from build123d import *

# Parameters (mm, degrees)
SKETCH_1_W           = 30
SKETCH_1_H           = 25
SKETCH_1_W_2         = 26
SKETCH_1_H_2         = 21
EXTRUDE_1_DEPTH      = 510
CUT_EXTRUDE_4_REACH  = 512.833
SKETCH_7_R           = 2.05
CUT_EXTRUDE_7_DEPTH  = 512.03449003
SKETCH_9_R           = 2.05
CUT_EXTRUDE_9_DEPTH  = 10
SKETCH_10_R          = 4
CUT_EXTRUDE_10_DEPTH = 10
SKETCH_11_R          = 2.05
CUT_EXTRUDE_11_DEPTH = 52
SKETCH_12_W          = 15
SKETCH_12_H          = 25
CUT_EXTRUDE_12_DEPTH = 512.03449003
CUT_EXTRUDE_13_REACH = 512.833
SKETCH_5_R           = 1.55


with BuildPart() as part:
    # 草图1 → 凸台-拉伸1 (new body)
    with BuildSketch(Plane.XY):
        Rectangle(SKETCH_1_W, SKETCH_1_H)
        Rectangle(SKETCH_1_W_2, SKETCH_1_H_2, mode=Mode.SUBTRACT)
    extrude(amount=EXTRUDE_1_DEPTH)

    # 草图4 → 切除-拉伸4 (cut, up to next)
    with BuildSketch(Plane.XZ.offset(12.5), mode=Mode.PRIVATE) as cut_extrude_4_sk1:
        with BuildLine():
            Line((-7.5, 40), (-7.5, 60))
            ThreePointArc((-7.5, 60), (0, 67.5), (7.5, 60))
            Line((7.5, 60), (7.5, 40))
            ThreePointArc((7.5, 40), (0, 32.5), (-7.5, 40))
        make_face()
    cut_extrude_4_tool1 = extrude(cut_extrude_4_sk1.sketch, amount=-CUT_EXTRUDE_4_REACH, mode=Mode.PRIVATE) & part.part
    # 草图4 → 切除-拉伸4 (cut, up to next)
    with BuildSketch(Plane.XZ.offset(12.5), mode=Mode.PRIVATE) as cut_extrude_4_sk2:
        with BuildLine():
            Line((-7.5, 190), (-7.5, 210))
            ThreePointArc((-7.5, 210), (0, 217.5), (7.5, 210))
            Line((7.5, 210), (7.5, 190))
            ThreePointArc((7.5, 190), (0, 182.5), (-7.5, 190))
        make_face()
    cut_extrude_4_tool2 = extrude(cut_extrude_4_sk2.sketch, amount=-CUT_EXTRUDE_4_REACH, mode=Mode.PRIVATE) & part.part
    # 草图4 → 切除-拉伸4 (cut, up to next)
    with BuildSketch(Plane.XZ.offset(12.5), mode=Mode.PRIVATE) as cut_extrude_4_sk3:
        with BuildLine():
            Line((-7.5, 340), (-7.5, 360))
            ThreePointArc((-7.5, 360), (0, 367.5), (7.5, 360))
            Line((7.5, 360), (7.5, 340))
            ThreePointArc((7.5, 340), (0, 332.5), (-7.5, 340))
        make_face()
    cut_extrude_4_tool3 = extrude(cut_extrude_4_sk3.sketch, amount=-CUT_EXTRUDE_4_REACH, mode=Mode.PRIVATE) & part.part
    add(cut_extrude_4_tool1.solids().sort_by_distance((0, -12.5, 50))[0], mode=Mode.SUBTRACT)
    add(cut_extrude_4_tool2.solids().sort_by_distance((0, -12.5, 200))[0], mode=Mode.SUBTRACT)
    add(cut_extrude_4_tool3.solids().sort_by_distance((0, -12.5, 350))[0], mode=Mode.SUBTRACT)

    # 草图7 → 切除-拉伸7 (cut, through all)
    with BuildSketch(Plane(origin=(15, 0, 0), x_dir=(0, 0, -1), z_dir=(1, 0, 0))):
        with Locations((-30, -5.5)):
            Circle(SKETCH_7_R)
        with Locations((-50, 4.5)):
            Circle(SKETCH_7_R)
        with Locations((-70, -5.5)):
            Circle(SKETCH_7_R)
    extrude(amount=-CUT_EXTRUDE_7_DEPTH, mode=Mode.SUBTRACT)

    # 草图9 → 切除-拉伸9 (cut)
    with BuildSketch(Plane.XZ.offset(12.5)):
        with Locations(Location((0, 480, 0), (0, 0, 270))):
            Circle(SKETCH_9_R)
        with Locations(Location((0, 500, 0), (0, 0, 270))):
            Circle(SKETCH_9_R)
        with Locations(Location((0, 440, 0), (0, 0, 90))):
            Circle(SKETCH_9_R)
        with Locations(Location((0, 460, 0), (0, 0, 90))):
            Circle(SKETCH_9_R)
    extrude(amount=-CUT_EXTRUDE_9_DEPTH, mode=Mode.SUBTRACT)

    # 草图10 → 切除-拉伸10 (cut)
    with BuildSketch(Plane(origin=(0, 12.5, 0), x_dir=(1, 0, 0), z_dir=(0, 1, 0))):
        with Locations(Location((0, -500, 0), (0, 0, 270))):
            Circle(SKETCH_10_R)
        with Locations(Location((0, -480, 0), (0, 0, 270))):
            Circle(SKETCH_10_R)
        with Locations(Location((0, -460, 0), (0, 0, 90))):
            Circle(SKETCH_10_R)
        with Locations(Location((0, -440, 0), (0, 0, 90))):
            Circle(SKETCH_10_R)
    extrude(amount=-CUT_EXTRUDE_10_DEPTH, mode=Mode.SUBTRACT)

    # 草图11 → 切除-拉伸11 (cut)
    with BuildSketch(Plane.ZY.offset(15)):
        with Locations((480, 7)):
            Circle(SKETCH_11_R)
        with Locations((500, 7)):
            Circle(SKETCH_11_R)
        with Locations((480, -7)):
            Circle(SKETCH_11_R)
        with Locations((500, -7)):
            Circle(SKETCH_11_R)
        with Locations((110, 7)):
            Circle(SKETCH_11_R)
        with Locations((130, 7)):
            Circle(SKETCH_11_R)
        with Locations((110, -7)):
            Circle(SKETCH_11_R)
        with Locations((130, -7)):
            Circle(SKETCH_11_R)
    extrude(amount=-CUT_EXTRUDE_11_DEPTH, mode=Mode.SUBTRACT)

    # 草图12 → 切除-拉伸12 (cut, through all)
    with BuildSketch(Plane.ZY.offset(15)):
        with Locations((7.5, 0)):
            Rectangle(SKETCH_12_W, SKETCH_12_H)
    extrude(amount=-CUT_EXTRUDE_12_DEPTH, mode=Mode.SUBTRACT)

    # 草图5 → 切除-拉伸13 (cut, up to next)
    with BuildSketch(Plane(origin=(0, 12.5, 0), x_dir=(1, 0, 0), z_dir=(0, 1, 0)), mode=Mode.PRIVATE) as cut_extrude_13_sk1:
        with Locations(Location((-10, -43, 0), (0, 0, 270))):
            Circle(SKETCH_5_R)
    cut_extrude_13_tool1 = extrude(cut_extrude_13_sk1.sketch, amount=-CUT_EXTRUDE_13_REACH, mode=Mode.PRIVATE) & part.part
    # 草图5 → 切除-拉伸13 (cut, up to next)
    with BuildSketch(Plane(origin=(0, 12.5, 0), x_dir=(1, 0, 0), z_dir=(0, 1, 0)), mode=Mode.PRIVATE) as cut_extrude_13_sk2:
        with Locations(Location((10, -43, 0), (0, 0, 270))):
            Circle(SKETCH_5_R)
    cut_extrude_13_tool2 = extrude(cut_extrude_13_sk2.sketch, amount=-CUT_EXTRUDE_13_REACH, mode=Mode.PRIVATE) & part.part
    # 草图5 → 切除-拉伸13 (cut, up to next)
    with BuildSketch(Plane(origin=(0, 12.5, 0), x_dir=(1, 0, 0), z_dir=(0, 1, 0)), mode=Mode.PRIVATE) as cut_extrude_13_sk3:
        with Locations(Location((-10, -63, 0), (0, 0, 270))):
            Circle(SKETCH_5_R)
    cut_extrude_13_tool3 = extrude(cut_extrude_13_sk3.sketch, amount=-CUT_EXTRUDE_13_REACH, mode=Mode.PRIVATE) & part.part
    # 草图5 → 切除-拉伸13 (cut, up to next)
    with BuildSketch(Plane(origin=(0, 12.5, 0), x_dir=(1, 0, 0), z_dir=(0, 1, 0)), mode=Mode.PRIVATE) as cut_extrude_13_sk4:
        with Locations(Location((10, -63, 0), (0, 0, 270))):
            Circle(SKETCH_5_R)
    cut_extrude_13_tool4 = extrude(cut_extrude_13_sk4.sketch, amount=-CUT_EXTRUDE_13_REACH, mode=Mode.PRIVATE) & part.part
    # 草图5 → 切除-拉伸13 (cut, up to next)
    with BuildSketch(Plane(origin=(0, 12.5, 0), x_dir=(1, 0, 0), z_dir=(0, 1, 0)), mode=Mode.PRIVATE) as cut_extrude_13_sk5:
        with Locations(Location((-10, -193, 0), (0, 0, 270))):
            Circle(SKETCH_5_R)
    cut_extrude_13_tool5 = extrude(cut_extrude_13_sk5.sketch, amount=-CUT_EXTRUDE_13_REACH, mode=Mode.PRIVATE) & part.part
    # 草图5 → 切除-拉伸13 (cut, up to next)
    with BuildSketch(Plane(origin=(0, 12.5, 0), x_dir=(1, 0, 0), z_dir=(0, 1, 0)), mode=Mode.PRIVATE) as cut_extrude_13_sk6:
        with Locations(Location((-10, -213, 0), (0, 0, 270))):
            Circle(SKETCH_5_R)
    cut_extrude_13_tool6 = extrude(cut_extrude_13_sk6.sketch, amount=-CUT_EXTRUDE_13_REACH, mode=Mode.PRIVATE) & part.part
    # 草图5 → 切除-拉伸13 (cut, up to next)
    with BuildSketch(Plane(origin=(0, 12.5, 0), x_dir=(1, 0, 0), z_dir=(0, 1, 0)), mode=Mode.PRIVATE) as cut_extrude_13_sk7:
        with Locations(Location((10, -193, 0), (0, 0, 270))):
            Circle(SKETCH_5_R)
    cut_extrude_13_tool7 = extrude(cut_extrude_13_sk7.sketch, amount=-CUT_EXTRUDE_13_REACH, mode=Mode.PRIVATE) & part.part
    # 草图5 → 切除-拉伸13 (cut, up to next)
    with BuildSketch(Plane(origin=(0, 12.5, 0), x_dir=(1, 0, 0), z_dir=(0, 1, 0)), mode=Mode.PRIVATE) as cut_extrude_13_sk8:
        with Locations(Location((10, -213, 0), (0, 0, 270))):
            Circle(SKETCH_5_R)
    cut_extrude_13_tool8 = extrude(cut_extrude_13_sk8.sketch, amount=-CUT_EXTRUDE_13_REACH, mode=Mode.PRIVATE) & part.part
    # 草图5 → 切除-拉伸13 (cut, up to next)
    with BuildSketch(Plane(origin=(0, 12.5, 0), x_dir=(1, 0, 0), z_dir=(0, 1, 0)), mode=Mode.PRIVATE) as cut_extrude_13_sk9:
        with Locations(Location((-10, -343, 0), (0, 0, 270))):
            Circle(SKETCH_5_R)
    cut_extrude_13_tool9 = extrude(cut_extrude_13_sk9.sketch, amount=-CUT_EXTRUDE_13_REACH, mode=Mode.PRIVATE) & part.part
    # 草图5 → 切除-拉伸13 (cut, up to next)
    with BuildSketch(Plane(origin=(0, 12.5, 0), x_dir=(1, 0, 0), z_dir=(0, 1, 0)), mode=Mode.PRIVATE) as cut_extrude_13_sk10:
        with Locations(Location((-10, -363, 0), (0, 0, 270))):
            Circle(SKETCH_5_R)
    cut_extrude_13_tool10 = extrude(cut_extrude_13_sk10.sketch, amount=-CUT_EXTRUDE_13_REACH, mode=Mode.PRIVATE) & part.part
    # 草图5 → 切除-拉伸13 (cut, up to next)
    with BuildSketch(Plane(origin=(0, 12.5, 0), x_dir=(1, 0, 0), z_dir=(0, 1, 0)), mode=Mode.PRIVATE) as cut_extrude_13_sk11:
        with Locations(Location((10, -343, 0), (0, 0, 270))):
            Circle(SKETCH_5_R)
    cut_extrude_13_tool11 = extrude(cut_extrude_13_sk11.sketch, amount=-CUT_EXTRUDE_13_REACH, mode=Mode.PRIVATE) & part.part
    # 草图5 → 切除-拉伸13 (cut, up to next)
    with BuildSketch(Plane(origin=(0, 12.5, 0), x_dir=(1, 0, 0), z_dir=(0, 1, 0)), mode=Mode.PRIVATE) as cut_extrude_13_sk12:
        with Locations(Location((10, -363, 0), (0, 0, 270))):
            Circle(SKETCH_5_R)
    cut_extrude_13_tool12 = extrude(cut_extrude_13_sk12.sketch, amount=-CUT_EXTRUDE_13_REACH, mode=Mode.PRIVATE) & part.part
    add(cut_extrude_13_tool1.solids().sort_by_distance((-10, 12.5, 43))[0], mode=Mode.SUBTRACT)
    add(cut_extrude_13_tool2.solids().sort_by_distance((10, 12.5, 43))[0], mode=Mode.SUBTRACT)
    add(cut_extrude_13_tool3.solids().sort_by_distance((-10, 12.5, 63))[0], mode=Mode.SUBTRACT)
    add(cut_extrude_13_tool4.solids().sort_by_distance((10, 12.5, 63))[0], mode=Mode.SUBTRACT)
    add(cut_extrude_13_tool5.solids().sort_by_distance((-10, 12.5, 193))[0], mode=Mode.SUBTRACT)
    add(cut_extrude_13_tool6.solids().sort_by_distance((-10, 12.5, 213))[0], mode=Mode.SUBTRACT)
    add(cut_extrude_13_tool7.solids().sort_by_distance((10, 12.5, 193))[0], mode=Mode.SUBTRACT)
    add(cut_extrude_13_tool8.solids().sort_by_distance((10, 12.5, 213))[0], mode=Mode.SUBTRACT)
    add(cut_extrude_13_tool9.solids().sort_by_distance((-10, 12.5, 343))[0], mode=Mode.SUBTRACT)
    add(cut_extrude_13_tool10.solids().sort_by_distance((-10, 12.5, 363))[0], mode=Mode.SUBTRACT)
    add(cut_extrude_13_tool11.solids().sort_by_distance((10, 12.5, 343))[0], mode=Mode.SUBTRACT)
    add(cut_extrude_13_tool12.solids().sort_by_distance((10, 12.5, 363))[0], mode=Mode.SUBTRACT)


solid = part.part
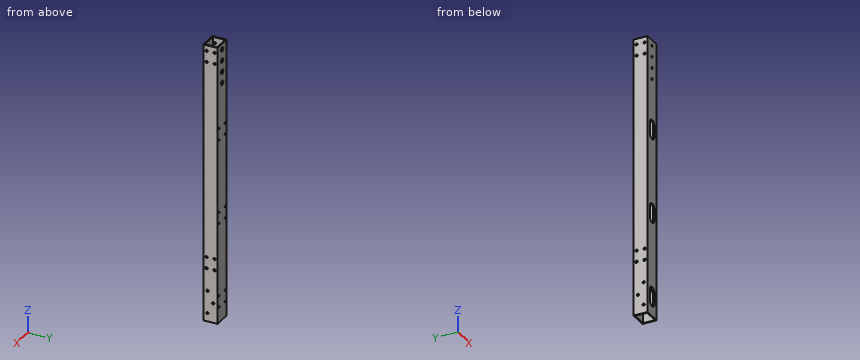
Geometry: final body of the model. Coordinates: model frame, mm. Give positions to 0.01 mm unless a question says otherwise; leave off trailing zeros. Write each loop counter-clockwise with the first axis right and the second up, starting at its lowest first coordinate (ties: lowest second). Pieces come first, ordered by that corner, then holes.
(1) First-contact query: P1, Ø6.5, axis at x = 0, z = 460, coming from the +Y side; P2, Ø2.5, axis at y = -7, z = 480, coming from the +X side. Flat tips, straight axial feed; report the tip coordinate or a pass-through.
(2) Cut plane A-A, the plane z = 273.5. Return loops of the section in (x, y), then the cut area to 3 significant figures.
(3) Ray query, line 1 (X direction, y = 11.35, z = 363); line 2 (Y direction, x = -13.9, z = 110); line 3 (X direction, y = 1.75, z = 138.5). Return the intervals inside material, ascending.
Values follow:
1. P1: stops at y = -10.5
1. P2: passes through
2. outline: (-15, -12.5) - (15, -12.5) - (15, 12.5) - (-15, 12.5) - close; hole (-13, -10.5) - (13, -10.5) - (13, 10.5) - (-13, 10.5) - close
2. area: 204 mm2
3. line 1: x = -15 to -11.55, -8.45 to 8.45, 11.55 to 15
3. line 2: y = -12.5 to -9.05, -4.95 to 4.95, 9.05 to 12.5
3. line 3: x = -15 to -13, 13 to 15
